from build123d import *

# Parameters (mm, degrees)
SKETCH005_W  = 14.63643
SKETCH005_H  = 13
PAD004_DEPTH = 5
SKETCH_W     = 35
SKETCH_H     = 13
PAD_DEPTH    = 5
SKETCH003_R  = 3.3
PAD003_DEPTH = 13


with BuildPart() as pad004:
    # Sketch005 → Pad004 (new body)
    with BuildSketch(Plane(origin=(0, 0, 0), x_dir=(1, 0, 0), z_dir=(0, 0, -1))):
        Rectangle(SKETCH005_W, SKETCH005_H)
    extrude(amount=PAD004_DEPTH)


with BuildPart() as fusion:
    # Sketch → Pad (new body)
    with BuildSketch(Plane.XY):
        Rectangle(SKETCH_W, SKETCH_H)
    extrude(amount=PAD_DEPTH)

    # Sketch003 → Pad003 (new body)
    with BuildSketch(Plane.XZ.offset(6.5)):
        with Locations((17.683945, 2.483897)):
            Circle(SKETCH003_R)
        with Locations((-17.683945, 2.483897)):
            Circle(SKETCH003_R)
    extrude(amount=-PAD003_DEPTH)

    # Fusion: union Pad004
    add(pad004.part)


solid = fusion.part
Input: part model. Units: mm. Frame: model coordinates. A direction names the side the tool comes from. Coordinates: 2 decimals unless noted, no trailing zeros. Order: outer loops, then holes, each group sorted by start corner. A loop starts at its lowest first (then second) coordinate and runs counter-clockwise, first axis right, second up.
1. Cut plane C-C, the plane z = -1.5. Return loops of the section in (x, y), plus the area to 3 significant figures.
Checked values:
outline: (-7.32, -6.5) - (7.32, -6.5) - (7.32, 6.5) - (-7.32, 6.5) - close
area: 190 mm2
2. Ray query, line 1 along X through (y, z) = (-0.5, -4.5); line 2 along Z through (x, y) = (13.5, -5); line 3 along Z through (x, y) = (-4.5, -4.5). Return the intervals inside material, ascending.
Checked values:
line 1: x = -7.32 to 7.32
line 2: z = 0 to 5
line 3: z = -5 to 5
3. Contact query for flat-ended pins moving along their axis: P1, Ø1.5, axis at y = -4, z = 0.5, coming from the -X side; P2, Ø3, axis at x = 12, z = -2.5, coming from the -Y side; P3, Ø5, axis at x = -13.5, y = -3.5, coming from the +Z side; P4, Ø5.5, axis at y = -0.5, z = -2, coming from the -X side. Output: stop coordinate, or through.
Checked values:
P1: stops at x = -20.74
P2: passes through
P3: stops at z = 5.32
P4: stops at x = -20.49
4. Cut plane A-A, the plane y = 5.25. Return loops of the section in (x, z), plus the area to 3 significant figures.
Checked values:
outline: (-15.55, 5) arc R3.3 ccw (long way) to (-15.51, 0) - (-7.32, 0) - (-7.32, -5) - (7.32, -5) - (7.32, 0) - (15.51, 0) arc R3.3 ccw (long way) to (15.55, 5) - close
area: 289 mm2
5. Draft query along X for faces 1 (the cylindrical face through (-20.983, -0.091, 2.565)), 2 (the flat face through (0, 0, 5)), 3 (the flat face through (0, 0, -5)). Return one class per face: +X half, -X half, draft (parallel to the pull), parting line (faces both ways), or undercut.
Checked values:
face 1: undercut
face 2: undercut
face 3: draft
6. Access query for faces 4 (the flat face through (-11, 0, 0)), 5 (the flat face through (0, 6.5, 2)). Directions: +Z, -Z, +X, -X, +Y, -Y. A direction counts if a zero-diameter tool reaches every point of the face in a straight line with its end or side. Return the directions, or none.
Checked values:
face 4: -Z, +Y, -Y
face 5: +Z, -Z, +X, -X, +Y
7. Cut plane B-B, the plane x = 12.5. Return loops of the section in (y, z), plus the area to 3 significant figures.
Checked values:
outline: (-6.5, 0) - (6.5, 0) - (6.5, 5) - (-6.5, 5) - close
area: 65.0 mm2
